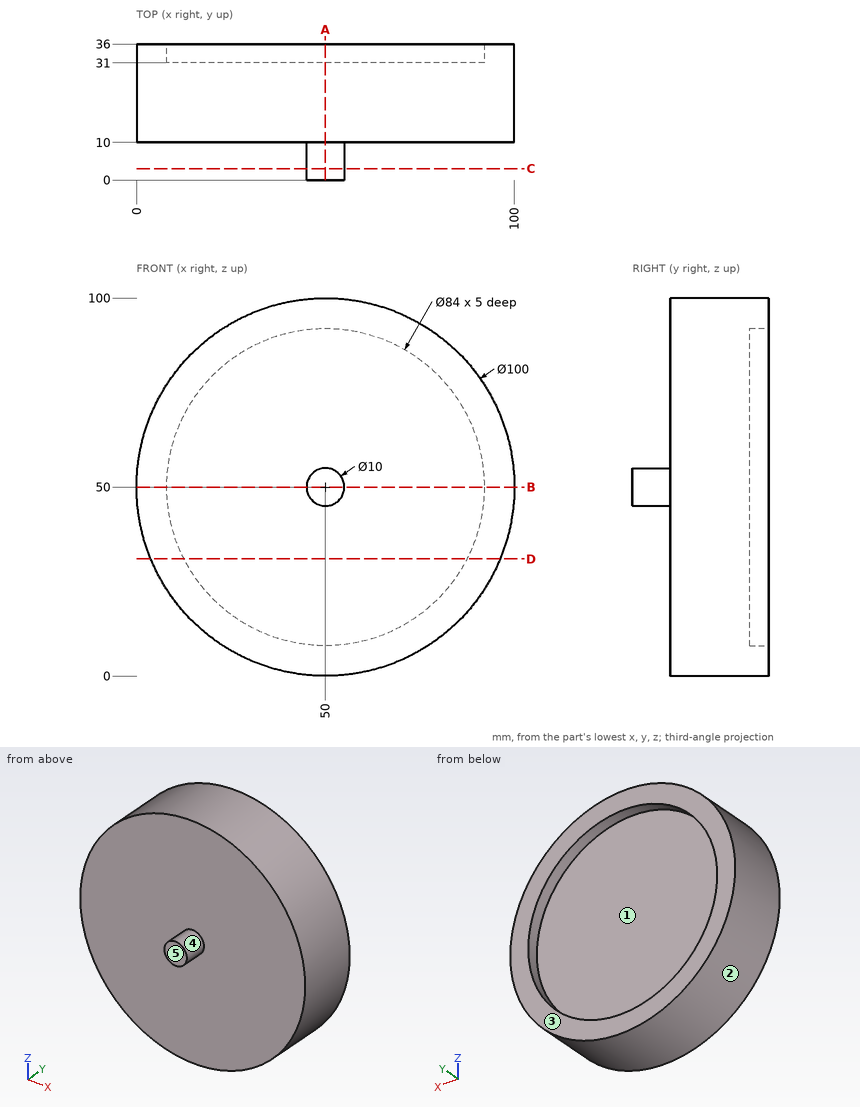
Job drawing, mm, ordinate dimensions from the low corner. One solid piece. A direction names the side the tool comes from. Round coordinates to 2 decimals unless told otherwise and drop trailing zeros. Loops run counter-clockwise (first coordinate to the right, second up) from the corner with the lowest first, then second, coordinate; pieces in that order, holes last. Notation, with made-up numbers: (22.5, 43.25) -> (30.5, 43.25) arc R24 cw to (30.5, 79.25) -> close; hole circle Ø3 at (76.5, -9). An arc over 180 degrees is marked (long way). Use CSV: the item, a comma, the result in double quotes. Start each with the question number.
Q1. Saw through at A-A on x = 50. Give the cut face in (y, z), and give its area (3 significant figures).
Q2. Saw through at C-C on y = 3. Give the cut face in (x, z), and give its area (3 significant figures).
Q3. Flat gauge pins, fed straight in: pin 1 Ø8 at (y, z) = (14.5, 39) entering from +X; pin 2 Ø6 at (x, y) = (69, 25) entering from -Z; pin 3 Ø5 at (y, z) = (17, 85.5) entering from -X. Where does each tip first touch, or does it go through?
Q4. Drill centre lines: L1, parallel to Z at x = 50, y = 34.85; L2, parallel to Y at x = 91, z = 26. Where is each one in solid material? Low to high.
Q5. Saw through at B-B on z = 50. Give the cut face in (x, y), and give its area (3 significant figures).
Q6. Mould opens along Z. For the marked faces 1, 2 and 3 say: +Z half, -Z half, draft (parallel to the pull), parting line (faces both ways), or undercut.
Q7. Saw through at D-D on z = 31. Give the cut face in (x, y).
Q8. Which spindle directions (+Z, -Z, +X, -X, +Y, -Y) get a long thin tool onto all of the face, cutting with end or side? Do the marked faces 4 and 5. Say none if no direction does.
Solutions:
1,outline,"(0, 45) -> (10, 45) -> (10, 0) -> (36, 0) -> (36, 8) -> (31, 8) -> (31, 92) -> (36, 92) -> (36, 100) -> (10, 100) -> (10, 55) -> (0, 55) -> close"
1,area,"2,280 mm^2"
2,outline,"circle Ø10 at (50, 50)"
2,area,"78.5 mm^2"
3,pin 1,"stops at x = 99.51"
3,pin 2,"stops at z = 2.63"
3,pin 3,"stops at x = 12.44"
4,L1,"z = 0 to 8, 92 to 100"
4,L2,"y = 10 to 36"
5,outline,"(0, 10) -> (45, 10) -> (45, 0) -> (55, 0) -> (55, 10) -> (100, 10) -> (100, 36) -> (92, 36) -> (92, 31) -> (8, 31) -> (8, 36) -> (0, 36) -> close"
5,area,"2,280 mm^2"
6,face 1,"undercut"
6,face 2,"parting line"
6,face 3,"draft"
7,outline,"(3.75, 10) -> (96.25, 10) -> (96.25, 36) -> (87.46, 36) -> (87.46, 31) -> (12.54, 31) -> (12.54, 36) -> (3.75, 36) -> close"
8,face 4,"-Y"
8,face 5,"+Z, -Z, +X, -X, -Y"
